Part model, mm, in its own coordinate system. Coordinates: 2 decimals unless noted, no trailing zeros. Write each loop counter-clockwise with the first axis right and the second up, starting at its lowest first coordinate (ties: lowest second). Pieces come first, ordered by that corner, then holes. Notation, with made-up numbers: (19.5, 63.5) -> (27.5, 63.5) arc R26 cw to (27.5, 82.5) -> close; hole circle Ø6 at (-14.5, -4.5). An arc over 180 degrees is marked (long way). One line per question, with ' | ' between items. Start each with the question number.
Item 1: Saw through at C-C (y = -420). List the corners of the cut face in (x, z), and give its area (3 significant figures).
Item 2: Pin check, flat tip, straight feed: pin 1 (2 mm diameter, centred on y = -263.5, z = 2.5, fed in from +X). Stop position of the tip, or through.
Item 3: Two-plate mould, pull along Y, no slides. Class faces 1 (the cylindrical face through (-2.38, -410.74, 2.96)), 2 (the flat face through (-1, -189, 6)), 3 (the cylindrical face through (-14.985, 0.66, 2.958)), 4 (the flat face through (67.348, -205.327, 2.958)): pulls with the +Y half, pulls with the -Y half, needs draft (parallel to the pull), parting line crosses it, or undercut.
Item 4: Saw through at A-A (x = 0). List the corners of the cut face in (y, z), and give its area (3 significant figures).
Item 5: Probe probe 1 along Y at (x, z) = (0, 3.35); probe 2 along Y at (x, z) = (-9, 1.7); probe 3 along X at (y, z) = (17, 2.25). List the from-to ranges inside material, lowest first. Write a range as [from, to].
Item 6: Saw through at B-B (z = 1.65). Count the separate pieces of the cut face and the enclosed holes in it, and give its area (3 significant figures).
Item 7: Saw through at D-D (x = -38). List the corners of the cut face in (y, z), and give its area (3 significant figures).
from build123d import *

# Parameters (mm, degrees)
SKETCH_1_R          = 15
SKETCH_1_R_2        = 11
EXTRUDE_1_DEPTH     = 6
SKETCH_2_R          = 1.25
CUT_EXTRUDE_1_DEPTH = 10


with BuildPart() as part:
    # 草图1 → 凸台-拉伸1 (new body)
    with BuildSketch(Plane.XY):
        with BuildLine():
            Line((-74.947247073, -2.8125), (-59.957797658, -402.25))
            ThreePointArc((-59.957797658, -402.25), (0, -460), (59.957797658, -402.25))
            Line((59.957797658, -402.25), (74.947247073, -2.8125))
            ThreePointArc((74.947247073, -2.8125), (0, 75), (-74.947247073, -2.8125))
        make_face()
        Circle(SKETCH_1_R, mode=Mode.SUBTRACT)
        with Locations((0, -400)):
            Circle(SKETCH_1_R_2, mode=Mode.SUBTRACT)
    extrude(amount=EXTRUDE_1_DEPTH)

    # 草图2 → 切除-拉伸1 (cut, symmetric)
    with BuildSketch(Plane.XY.offset(6)):
        with Locations((13.980630511, 16.661466638)):
            Circle(SKETCH_2_R)
        with Locations((21.75, 0)):
            Circle(SKETCH_2_R)
        with Locations((13.980630511, -16.661466638)):
            Circle(SKETCH_2_R)
        with Locations((-13.980630511, 16.661466638)):
            Circle(SKETCH_2_R)
        with Locations((-21.75, 0)):
            Circle(SKETCH_2_R)
        with Locations((-13.980630511, -16.661466638)):
            Circle(SKETCH_2_R)
    extrude(amount=CUT_EXTRUDE_1_DEPTH, both=True, mode=Mode.SUBTRACT)


solid = part.part
From the geometry:
1) outline: (-56.57, 0) -> (56.57, 0) -> (56.57, 6) -> (-56.57, 6) -> close | area: 679 mm2
2) pin 1: x = 65.2
3) face 1: undercut | face 2: needs draft | face 3: undercut | face 4: pulls with the -Y half
4) outline: (-460, 0) -> (-411, 0) -> (-411, 6) -> (-460, 6) -> close; (-389, 0) -> (-15, 0) -> (-15, 6) -> (-389, 6) -> close; (15, 0) -> (75, 0) -> (75, 6) -> (15, 6) -> close | area: 2,900 mm2
5) probe 1: [-460, -411], [-389, -15], [15, 75] | probe 2: [-459.32, -406.32], [-393.68, -12], [12, 74.46] | probe 3: [-73.05, -15.18], [-12.78, 12.78], [15.18, 73.05]
6) separate pieces: 1 | enclosed holes: 8 | area: 67,400 mm2
7) outline: (-446.43, 0) -> (64.66, 0) -> (64.66, 6) -> (-446.43, 6) -> close | area: 3,070 mm2
